Verification items for this drawing (mm, ordinates from the low corner). A direction names the side the tool comes from. Give positions to 0.01 mm unless a question says otherwise; leave off trailing zeros. Order: outer loops, then holes, each group sorted by start corner. A loop starts at its lowest first (then second) coordinate and runs counter-clockwise, first axis right, second up.
(1) Mould release check, pull along X, two halves, no side actions. Record for the marked faces 3, 4 and 5: pulls with the +X half, pulls with the -X half, needs draft (parallel to the pull), parting line crosses it, or undercut.
(2) Sectioned sample at B-B on y = 24.15. Record the cut outline in (x, z).
(3) Scan lines: L1, parallel to X at y = 0.5, z = 10; L2, parallel to Y at x = 8.65, z = 1.7; L3, parallel to Y at x = 39.65, z = 0.8. Record each from-to range of solid material in increasing order.
(4) Gauge pin test, flat ends, axial feed: pin 1 (12 mm diameter, centred on x = 13, y = 22.5, fed in from +Z); pin 2 (3 mm diameter, centred on x = 8.5, z = 10, fed in from +Y); pin 3 (4 mm diameter, centred on x = 14.15, z = 10, fed in from +Y). Record the tip position at first contact, or that the pin passes through.
(5) Sectioned sample at A-A on x = 39.65. Record the cut outline in (y, z), plus the area to 3 significant figures.
(6) Sectioned sample at D-D on x = 24.15. Record the cut outline in (y, z).
(7) Sectioned sample at C-C on z = 10. Record the cut outline in (x, y).
(8) Access from +Z, -Z, +X, -X, +Y, -Y to the whole of each face (thin tool, end or side, straight path). Record for the marked faces 1 and 2.
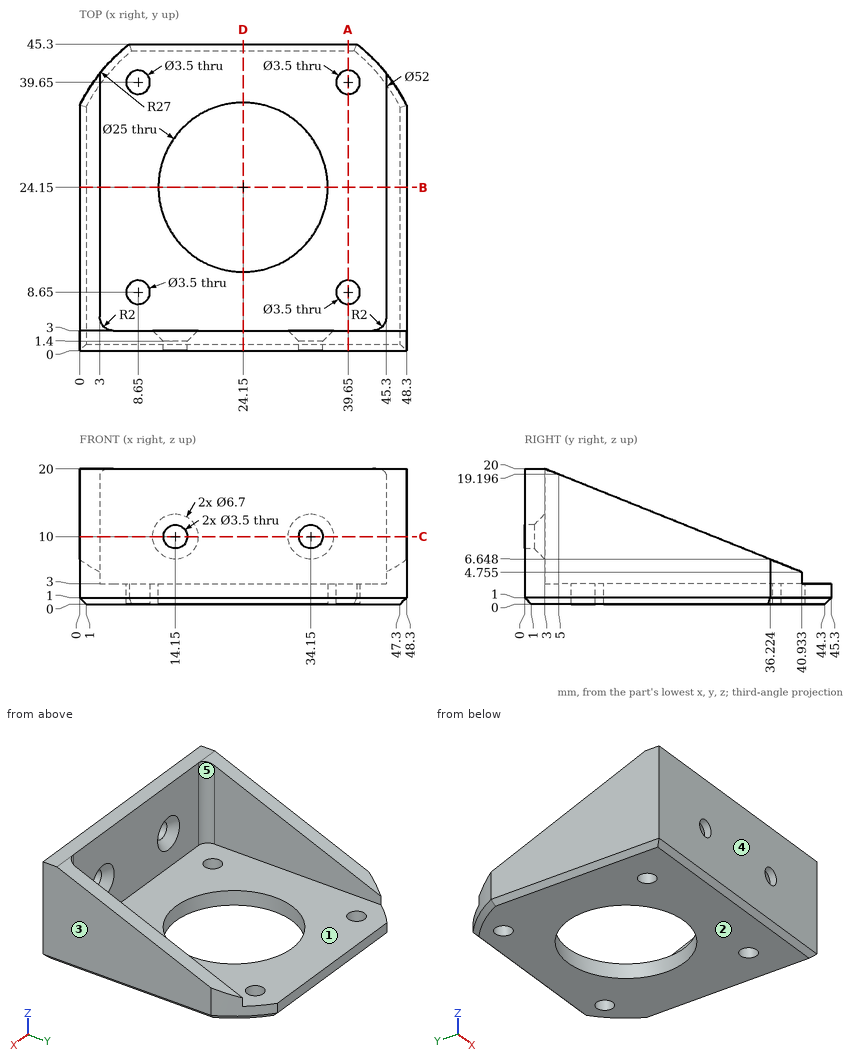
Ans:
1. face 3: pulls with the +X half
1. face 4: needs draft
1. face 5: undercut
2. outline: (0, 1) - (1, 0) - (11.65, 0) - (11.65, 3) - (3, 3) - (3, 11.5) - (0, 11.5) - close; (36.65, 0) - (47.3, 0) - (48.3, 1) - (48.3, 11.5) - (45.3, 11.5) - (45.3, 3) - (36.65, 3) - close
3. L1: x = 0 to 12.4, 15.9 to 32.4, 35.9 to 48.3
3. L2: y = 0 to 6.9, 10.4 to 37.9, 41.4 to 45.3
3. L3: y = 0.2 to 6.9, 10.4 to 37.9, 41.4 to 45.1
4. pin 1: stops at z = 3
4. pin 2: stops at y = 3
4. pin 3: stops at y = 1.65
5. outline: (0, 1) - (1, 0) - (6.9, 0) - (6.9, 3) - (3, 3) - (3, 20) - (0, 20) - close; (10.4, 0) - (37.9, 0) - (37.9, 3) - (10.4, 3) - close; (41.4, 0) - (44.3, 0) - (45.3, 1) - (45.3, 3) - (41.4, 3) - close
5. area: 165 mm2
6. outline: (0, 1) - (1, 0) - (11.65, 0) - (11.65, 3) - (3, 3) - (3, 20) - (0, 20) - close; (36.65, 0) - (44.3, 0) - (45.3, 1) - (45.3, 3) - (36.65, 3) - close
7. outline: (0, 0) - (12.4, 0) - (12.4, 1.4) - (10.8, 3) - (5, 3) arc R2 cw to (3, 5) - (3, 27.88) - (0, 27.88) - close; (15.9, 0) - (32.4, 0) - (32.4, 1.4) - (30.8, 3) - (17.5, 3) - (15.9, 1.4) - close; (35.9, 0) - (48.3, 0) - (48.3, 27.88) - (45.3, 27.88) - (45.3, 5) arc R2 cw to (43.3, 3) - (37.5, 3) - (35.9, 1.4) - close
8. face 1: +Z, +Y
8. face 2: -Z, +X, -X, +Y, -Y
